The listing builds one solid part. Answer for the finished solid, in the listing's coordinates (mm). Round coordinates to 2 decimals unless told otherwise and drop trailing zeros. Write each loop counter-clockwise with the first axis right and the second up, starting at its lowest first coordinate (ties: lowest second). Pieces come first, ordered by that corner, then holes. Notation, with made-up numbers: M 44,63 L 50,63 A17 ccw 50,80 Z; hole C 11.25,48.25 d8. An arc over 180 degrees is marked long. Answer as CSV lines item,"result". Start each with the question number.
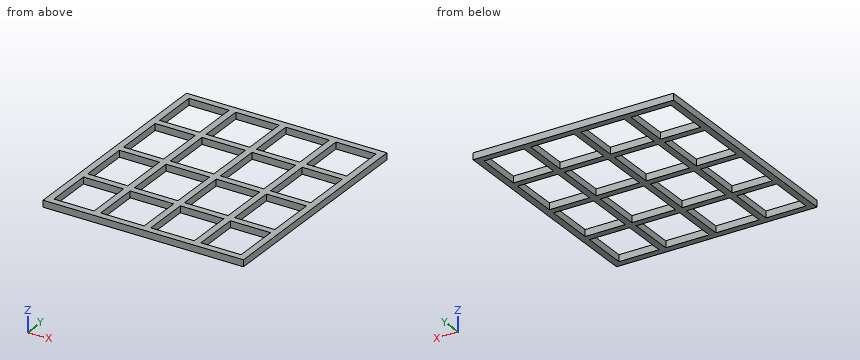
from build123d import *

# Parameters (mm, degrees)
F0_W     = 30
F0_H     = 35
F0_W_2   = 32.5
F0_H_2   = 37.5
F1_DEPTH = 5


with BuildPart() as f1:
    # F0 (on Top) → F1 (new body)
    with BuildSketch(Plane.XY):
        Polygon((-37.5, 85), (-75, 85), (-75, 42.5), (-75, 0), (-75, -42.5), (-75, -85), (-37.5, -85), (0, -85), (37.5, -85), (75, -85), (75, -42.5), (75, 0), (75, 42.5), (75, 85), (37.5, 85), (0, 85), align=None)
        with Locations((-55, -62.5)):
            Rectangle(F0_W, F0_H, mode=Mode.SUBTRACT)
        with Locations((-18.75, -62.5)):
            Rectangle(F0_W_2, F0_H, mode=Mode.SUBTRACT)
        with Locations((-55, -21.25)):
            Rectangle(F0_W, F0_H_2, mode=Mode.SUBTRACT)
        with Locations((-18.75, -21.25)):
            Rectangle(F0_W_2, F0_H_2, mode=Mode.SUBTRACT)
        with Locations((18.75, -62.5)):
            Rectangle(F0_W_2, F0_H, mode=Mode.SUBTRACT)
        with Locations((55, -62.5)):
            Rectangle(F0_W, F0_H, mode=Mode.SUBTRACT)
        with Locations((18.75, -21.25)):
            Rectangle(F0_W_2, F0_H_2, mode=Mode.SUBTRACT)
        with Locations((55, -21.25)):
            Rectangle(F0_W, F0_H_2, mode=Mode.SUBTRACT)
        with Locations((-55, 21.25)):
            Rectangle(F0_W, F0_H_2, mode=Mode.SUBTRACT)
        with Locations((-18.75, 21.25)):
            Rectangle(F0_W_2, F0_H_2, mode=Mode.SUBTRACT)
        with Locations((-55, 62.5)):
            Rectangle(F0_W, F0_H, mode=Mode.SUBTRACT)
        with Locations((-18.75, 62.5)):
            Rectangle(F0_W_2, F0_H, mode=Mode.SUBTRACT)
        with Locations((18.75, 21.25)):
            Rectangle(F0_W_2, F0_H_2, mode=Mode.SUBTRACT)
        with Locations((55, 21.25)):
            Rectangle(F0_W, F0_H_2, mode=Mode.SUBTRACT)
        with Locations((18.75, 62.5)):
            Rectangle(F0_W_2, F0_H, mode=Mode.SUBTRACT)
        with Locations((55, 62.5)):
            Rectangle(F0_W, F0_H, mode=Mode.SUBTRACT)
    extrude(amount=F1_DEPTH)


solid = f1.part
Q1. Find section C-C (z = 1.65). Count the separate pieces of the cut face and the enclosed holes in it, plus the area to 4 significant figures.
Q2. Straight lines are drawn through the part: L1, parallel to Y at x = -30.5, z = 2.4; L2, parallel to X at y = -60, z = 3.9. For each, find the intervals that lie inside material, in ascending order.
Q3. Find section B-B (y = 64). Determine the outline of the cut face in (x, z), plus the area to 3 significant figures.
Q4. Find section A-A (x = 21). Determine the outline of the cut face in (y, z).
Reported:
1,separate pieces,"1"
1,enclosed holes,"16"
1,area,"7,375 mm2"
2,L1,"y = -85 to -80, -45 to -40, -2.5 to 2.5, 40 to 45, 80 to 85"
2,L2,"x = -75 to -70, -40 to -35, -2.5 to 2.5, 35 to 40, 70 to 75"
3,outline,"M -75,0 L -70,0 L -70,5 L -75,5 Z; M -40,0 L -35,0 L -35,5 L -40,5 Z; M -2.5,0 L 2.5,0 L 2.5,5 L -2.5,5 Z; M 35,0 L 40,0 L 40,5 L 35,5 Z; M 70,0 L 75,0 L 75,5 L 70,5 Z"
3,area,"125 mm2"
4,outline,"M -85,0 L -80,0 L -80,5 L -85,5 Z; M -45,0 L -40,0 L -40,5 L -45,5 Z; M -2.5,0 L 2.5,0 L 2.5,5 L -2.5,5 Z; M 40,0 L 45,0 L 45,5 L 40,5 Z; M 80,0 L 85,0 L 85,5 L 80,5 Z"
